Verification items for the finished model (mm, model axes). Face numbers are marked on the shaded views. A direction names the side the tool comes from. Round coordinates to 2 decimals unless told otherwise and drop trailing zeros. Order: outer loops, then holes, each group sorted by start corner. A loop starts at its lowest first (then second) coordinate and runs counter-clockwise, first axis right, second up. Notation, with made-up numbers: M -27.75,-18 L 0.25,-18 A15 cw 0.25,4 Z; hole C 50.25,9.25 d3. An arc over 180 degrees is marked long. One line per item, written item: value. Start each with the question number.
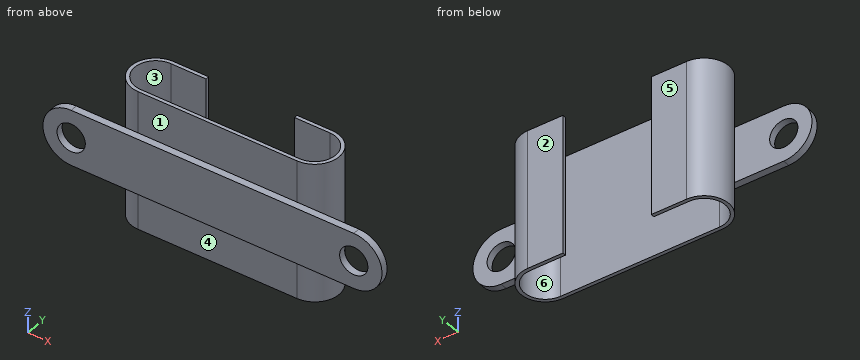
from build123d import *

# Parameters (mm, degrees)
BOSS_EXTRU_1_DEPTH      = 40
ENL_V_MAT_EXTRU_1_DEPTH = 66.977268813
ESQUISSE3_W             = 25.003743198
ESQUISSE3_H             = 40
ENL_V_MAT_EXTRU_2_DEPTH = 1
ESQUISSE4_R             = 4
BOSS_EXTRU_2_DEPTH      = 2


with BuildPart() as part:
    # Esquisse1 → Boss.-Extru.1 (new body)
    with BuildSketch(Plane.XY):
        with BuildLine():
            Line((0, 7), (45, 7))
            ThreePointArc((45, 7), (52, 0), (45, -7))
            Line((45, -7), (0, -7))
            ThreePointArc((0, -7), (-7, 0), (0, 7))
        make_face()
    extrude(amount=BOSS_EXTRU_1_DEPTH)

    # Esquisse2 → Enlèv. mat.-Extru.1 (cut, through all)
    with BuildSketch(Plane.XY.offset(40)):
        with BuildLine():
            Line((0, -6), (45, -6))
            ThreePointArc((45, -6), (51, 0), (45, 6))
            Line((45, 6), (0, 6))
            ThreePointArc((0, 6), (-6, 0), (0, -6))
        make_face()
    extrude(amount=-ENL_V_MAT_EXTRU_1_DEPTH, mode=Mode.SUBTRACT)

    # Esquisse3 → Enlèv. mat.-Extru.2 (cut)
    with BuildSketch(Plane(origin=(0, 7, 0), x_dir=(1, 0, 0), z_dir=(0, 1, 0))):
        with Locations((22.5, -20)):
            Rectangle(ESQUISSE3_W, ESQUISSE3_H)
    extrude(amount=-ENL_V_MAT_EXTRU_2_DEPTH, mode=Mode.SUBTRACT)

    # Esquisse4 → Boss.-Extru.2 (add)
    with BuildSketch(Plane(origin=(0, -7, 0), x_dir=(-1, 0, 0), z_dir=(0, -1, 0))):
        with BuildLine():
            Line((-62.5, -12), (17.5, -12))
            ThreePointArc((17.5, -12), (25.5, -20), (17.5, -28))
            Line((17.5, -28), (-62.5, -28))
            ThreePointArc((-62.5, -28), (-70.5, -20), (-62.5, -12))
        make_face()
        with Locations(Location((17.5, -20, 0), (0, 0, 90))):
            Circle(ESQUISSE4_R, mode=Mode.SUBTRACT)
        with Locations(Location((-62.5, -20, 0), (0, 0, 270))):
            Circle(ESQUISSE4_R, mode=Mode.SUBTRACT)
    extrude(amount=BOSS_EXTRU_2_DEPTH)


solid = part.part
1. Section check A-A (x = 43.5). Record the cut outline in (y, z).
2. Section check D-D (y = -3.75). Record the cut outline in (x, z), and give its area (3 significant figures).
3. Section check C-C (z = 5.5). Record the cut outline in (x, y).
4. Section check B-B (y = -8). Record the cut outline in (x, z).
5. Draft check along Y on the marked faces 1, 2 and 3. Enter one of: released by +Y, released by -Y, zero draft, split by the parting line, or undercut.
6. Tool access check on the marked faces 4, 5 and 6. Record the directions out of +Z, -Z, +X, -X, +Y, -Y that give a thin tool (end or side, any length) a straight path to the whole face; none if there is none.
7. Depth check by flat-ended pin: pin 1 (5 mm diameter, centred on x = 55.5, z = 20.5, fed in from +Y); pin 2 (4 mm diameter, centred on x = -6, z = 32, fed in from +Y); pin 3 (13 mm diameter, centred on x = 27, z = 34, fed in from -Y); pin 4 (12 mm diameter, centred on x = 24, z = 17.5, fed in from +Y). Enter the tip coordinate at first touch or a pass-through.
8. Scan lines: line 1 along X through (y, z) = (-7.7, 20); line 2 along X through (y, z) = (-0.25, 7.5); line 3 along Y through (x, z) = (38, 23.5). Record each from-to range of solid material in increasing order.
Geometry check:
1. outline: M -9,12 L -7,12 L -7,0 L -6,0 L -6,40 L -7,40 L -7,28 L -9,28 Z; M 6,0 L 7,0 L 7,40 L 6,40 Z
2. outline: M -5.91,0 L -4.68,0 L -4.68,40 L -5.91,40 Z; M 49.68,0 L 50.91,0 L 50.91,40 L 49.68,40 Z
2. area: 98.2 mm²
3. outline: M 0,-7 L 45,-7 A7 ccw 45,7 L 35,7 L 35,6 L 45,6 A6 cw 45,-6 L 0,-6 A6 cw 0,6 L 10,6 L 10,7 L 0,7 A7 ccw Z
4. outline: M -17.5,12 L 62.5,12 A8 ccw 62.5,28 L -17.5,28 A8 ccw Z; hole C -17.5,20 d8; hole C 62.5,20 d8
5. face 1: released by -Y
5. face 2: released by +Y
5. face 3: undercut
6. face 4: -Z, +X, -X, -Y
6. face 5: +Z, -Z, +X, -X, +Y
6. face 6: +Z, -Z
7. pin 1: stops at y = -7
7. pin 2: stops at y = 5.74
7. pin 3: stops at y = -9
7. pin 4: stops at y = -6
8. line 1: x = -25.5 to -21.5, -13.5 to 58.5, 66.5 to 70.5
8. line 2: x = -7 to -5.99, 50.99 to 52
8. line 3: y = -9 to -6, 6 to 7
